```python
from build123d import *

# Parameters (mm, degrees)
F0_R     = 28.575
F0_R_2   = 3.2639
F0_R_3   = 2.4892
F0_R_4   = 14.29512
F1_DEPTH = 6.35
F2_DEPTH = 19.05
F3_R     = 1.27


with BuildPart() as f1:
    # F0 (on Front) → F1 (new body)
    with BuildSketch(Plane.XZ):
        Circle(F0_R)
        with Locations((-11.90625, -20.6222299276)):
            Circle(F0_R_2, mode=Mode.SUBTRACT)
        with Locations((-20.611231405, -11.8872)):
            Circle(F0_R_3, mode=Mode.SUBTRACT)
        with Locations((0, -23.7871)):
            Circle(F0_R_3, mode=Mode.SUBTRACT)
        with Locations((11.90625, -20.6222299276)):
            Circle(F0_R_2, mode=Mode.SUBTRACT)
        with Locations((20.611231405, -11.8872)):
            Circle(F0_R_3, mode=Mode.SUBTRACT)
        with Locations((-23.8125, 0)):
            Circle(F0_R_2, mode=Mode.SUBTRACT)
        with Locations((-20.611231405, 11.9126)):
            Circle(F0_R_3, mode=Mode.SUBTRACT)
        with Locations((-11.90625, 20.6222299276)):
            Circle(F0_R_2, mode=Mode.SUBTRACT)
        Circle(F0_R_4, mode=Mode.SUBTRACT)
        with Locations((23.8125, 0)):
            Circle(F0_R_2, mode=Mode.SUBTRACT)
        with Locations((20.611231405, 11.9126)):
            Circle(F0_R_3, mode=Mode.SUBTRACT)
        with Locations((11.90625, 20.6222299276)):
            Circle(F0_R_2, mode=Mode.SUBTRACT)
        with Locations((0, 23.8125)):
            Circle(F0_R_3, mode=Mode.SUBTRACT)
        Circle(F0_R_4)
        Polygon((-7.6989658396, 0.0127), (-3.8494829198, 6.6802), (3.8494829198, 6.6802), (7.6989658396, 0.0127), (3.8494829198, -6.6548), (-3.8494829198, -6.6548), align=None, mode=Mode.SUBTRACT)
    extrude(amount=F1_DEPTH)

    # F0 (on Front) → F2 (join)
    with BuildSketch(Plane.XZ):
        Circle(F0_R_4)
        Polygon((-7.6989658396, 0.0127), (-3.8494829198, 6.6802), (3.8494829198, 6.6802), (7.6989658396, 0.0127), (3.8494829198, -6.6548), (-3.8494829198, -6.6548), align=None, mode=Mode.SUBTRACT)
    extrude(amount=F2_DEPTH)

    # F3
    f3_edges = [f1.edges().sort_by_distance(p)[0] for p in [
        (-28.575, -6.35, 0),
        (-14.29512, -19.05, 0),
        (-14.29512, -6.35, 0),
    ]]
    fillet(f3_edges, radius=F3_R)


solid = f1.part
```
Here's how the part is built. I have some questions about the finished solid (model axes, mm). Coordinates: 2 decimals unless noted, no trailing zeros. Loops run counter-clockwise (first coordinate to the right, second up) from the corner with the lowest first, then second, coordinate; pieces in that order, holes last. Notation, with made-up numbers: M 61.25,25 L 114.25,25 A26 cw 114.25,41 Z; hole C 2,-33.5 d1. An arc over 180 degrees is marked long. One line per item, written item: value.
1. Imagine slicing it at C-C (y = -1.75). State how many separate pieces and enclosed holes the cut face has, and give its area (3 significant figures).
Geometry says:
separate pieces: 1
enclosed holes: 13
area: 2,090 mm2
2. Imagine slicing it at B-B (y = -14.25). List the corners of the cut face in (x, z) for me.
Geometry says:
outline: C 0,0 d28.59; hole M -7.7,0.01 L -3.85,-6.65 L 3.85,-6.65 L 7.7,0.01 L 3.85,6.68 L -3.85,6.68 Z
3. Imagine slicing it at A-A (x = 0). List the corners of the cut face in (y, z) for me (3 decimals).
Geometry says:
outline: M -19.05,-13.025 A1.27 ccw -17.78,-14.295 L -7.62,-14.295 A1.27 cw -6.35,-15.565 L -6.35,-21.298 L 0,-21.298 L 0,-6.655 L -19.05,-6.655 Z; M -19.05,6.68 L 0,6.68 L 0,21.323 L -6.35,21.323 L -6.35,15.565 A1.27 cw -7.62,14.295 L -17.78,14.295 A1.27 ccw -19.05,13.025 Z; M -6.35,-27.305 A1.27 ccw -5.08,-28.575 L 0,-28.575 L 0,-26.276 L -6.35,-26.276 Z; M -6.35,26.302 L 0,26.302 L 0,28.575 L -5.08,28.575 A1.27 ccw -6.35,27.305 Z
4. Please list where these lines run through material, in increasing order: probe 1 along Z at (x, y) = (0, -2.5) (3 decimals); probe 2 along Z at (x, y) = (-21, -5.75); probe 3 along X at (y, z) = (-3, -19.5).
Geometry says:
probe 1: z = -28.575 to -26.276, -21.298 to -6.655, 6.68 to 21.323, 26.302 to 28.575
probe 2: z = -19.1 to -14.35, -9.43 to -1.66, 1.66 to 9.45, 14.37 to 19.1
probe 3: x = -20.89 to -14.97, -8.84 to 8.84, 14.97 to 20.89
5. Will these pins go through, and if not, where does the flat tip stop? pin 1 Ø4 at (y, z) = (-12.5, 13.5) entering from -X; pin 2 Ø8 at (x, z) = (20.61, -11.89) entering from -Y; pin 3 Ø5 at (x, z) = (-11.91, 20.62) entering from +Y; pin 4 Ø8.5 at (x, y) = (-1.5, -10) entering from -Z.
Geometry says:
pin 1: stops at x = -8.49
pin 2: stops at y = -6.35
pin 3: passes through
pin 4: stops at z = -28.35
6. Thinking about a two-plate mould opening in Z: for faces 1 (the cylindrical face through (-1.861, -12.629, 14.173)), 2 (the cylindrical face through (-27.073, -3.131, 0.144)), 3 (the flat face through (6, -19.05, -6)), 4 (the cylindrical face through (-0.54, -3.131, -26.217)), which applies, +Z half, -Z half, draft (parallel to the pull), parting line (faces both ways), or undercut?
Geometry says:
face 1: parting line
face 2: undercut
face 3: draft
face 4: undercut
